Source: CAD feature listing. Evaluate the final solid. Frame: model axes, mm. Give positions to 0.01 mm unless a question says otherwise; leave off trailing zeros. Write each loop counter-clockwise with the first axis right and the second up, starting at its lowest first coordinate (ties: lowest second). Pieces come first, ordered by that corner, then holes. Notation, with made-up numbers: (41, 60) -> (89, 60) arc R17 ccw to (89, 93) -> close; hole circle Ø10 at (0.5, 63). An arc over 180 degrees is marked (long way). Use a Markdown table: item, result. Add a question column.
```python
from build123d import *

# Parameters (mm, degrees)
CROQUIS1_R              = 1.5
CROQUIS1_W              = 3.2
CROQUIS1_H              = 10
CROQUIS1_W_2            = 23
CROQUIS1_H_2            = 12
CROQUIS1_W_3            = 10
CROQUIS1_H_3            = 3.2
SALIENTE_EXTRUIR1_DEPTH = 3


with BuildPart() as part:
    # Croquis1 → Saliente-Extruir1 (new body)
    with BuildSketch(Plane.XY):
        with BuildLine():
            Line((25, -46), (-25, -46))
            Line((-25, -46), (-25, 36))
            ThreePointArc((-25, 36), (-22.071067812, 43.071067812), (-15, 46))
            Line((-15, 46), (15, 46))
            ThreePointArc((15, 46), (22.071067812, 43.071067812), (25, 36))
            Line((25, 36), (25, -46))
        make_face()
        with Locations((0, 42)):
            Circle(CROQUIS1_R, mode=Mode.SUBTRACT)
        with Locations(Location((0, 24, 0), (0, 0, 180))):
            Circle(CROQUIS1_R, mode=Mode.SUBTRACT)
        with Locations((0, -14.4)):
            Circle(CROQUIS1_R, mode=Mode.SUBTRACT)
        with Locations((-20.6, 11)):
            Rectangle(CROQUIS1_W, CROQUIS1_H, mode=Mode.SUBTRACT)
        with Locations((-20.6, -11)):
            Rectangle(CROQUIS1_W, CROQUIS1_H, mode=Mode.SUBTRACT)
        with Locations((20.6, 11)):
            Rectangle(CROQUIS1_W, CROQUIS1_H, mode=Mode.SUBTRACT)
        with Locations((20.6, -11)):
            Rectangle(CROQUIS1_W, CROQUIS1_H, mode=Mode.SUBTRACT)
        with Locations((0, 33)):
            Rectangle(CROQUIS1_W_2, CROQUIS1_H_2, mode=Mode.SUBTRACT)
        with Locations((10, -14.4)):
            Rectangle(CROQUIS1_W_3, CROQUIS1_H_3, mode=Mode.SUBTRACT)
        with Locations((-10, -14.4)):
            Rectangle(CROQUIS1_W_3, CROQUIS1_H_3, mode=Mode.SUBTRACT)
    extrude(amount=SALIENTE_EXTRUIR1_DEPTH)


solid = part.part
```
(1) Cut plane B-B on y = 12. Return the cut outline in (x, z), then the cut area to 3 significant figures.
(2) First-contact query: pin 1 Ø1 at (x, z) = (16.5, 2.5) entering from +Y. Flat tip, straight axial feed; report the tip coordinate or a pass-through.
(3) Material intervals for L1, parallel to Y at x = 0, z = 0.9; L2, parallel to X at y = 14, z = 2.15; L3, parallel to Y at x = 5.5, z = 0.5, sorted ascending.
(4) Mould query, pull axis Y, two halves, no side actions, for faces 1 (the flat face through (-5, -14, 1)), 2 (the flat face through (0, -46, 1)). Classes: +Y half, -Y half, draft (parallel to the pull), parting line (faces both ways), or undercut.
(5) Cut plane C-C on y = 24. Return the cut outline in (x, z).
(6) Cut plane A-A on x = 2.5. Return the cut outline in (y, z), then the cut area to 3 significant figures.
(7) Cut plane D-D on y = -14.4. Return the cut outline in (x, z), then the cut area to 3 significant figures.
Output:
| question | item | result |
|---|---|---|
| 1 | outline | (-25, 0) -> (-22.2, 0) -> (-22.2, 3) -> (-25, 3) -> close; (-19, 0) -> (19, 0) -> (19, 3) -> (-19, 3) -> close; (22.2, 0) -> (25, 0) -> (25, 3) -> (22.2, 3) -> close |
| 1 | area | 131 mm^2 |
| 2 | pin 1 | y = 45.95 |
| 3 | L1 | -46 to -15.9, -12.9 to 22.5, 25.5 to 27, 39 to 40.5, 43.5 to 46 |
| 3 | L2 | -25 to -22.2, -19 to 19, 22.2 to 25 |
| 3 | L3 | -46 to -16, -12.8 to 27, 39 to 46 |
| 4 | face 1 | undercut |
| 4 | face 2 | -Y half |
| 5 | outline | (-25, 0) -> (-1.5, 0) -> (-1.5, 3) -> (-25, 3) -> close; (1.5, 0) -> (25, 0) -> (25, 3) -> (1.5, 3) -> close |
| 6 | outline | (-46, 0) -> (27, 0) -> (27, 3) -> (-46, 3) -> close; (39, 0) -> (46, 0) -> (46, 3) -> (39, 3) -> close |
| 6 | area | 240 mm^2 |
| 7 | outline | (-25, 0) -> (-22.2, 0) -> (-22.2, 3) -> (-25, 3) -> close; (-19, 0) -> (-15, 0) -> (-15, 3) -> (-19, 3) -> close; (-5, 0) -> (-1.5, 0) -> (-1.5, 3) -> (-5, 3) -> close; (1.5, 0) -> (5, 0) -> (5, 3) -> (1.5, 3) -> close; (15, 0) -> (19, 0) -> (19, 3) -> (15, 3) -> close; (22.2, 0) -> (25, 0) -> (25, 3) -> (22.2, 3) -> close |
| 7 | area | 61.8 mm^2 |
